Source: CAD feature listing. Evaluate the final solid. Frame: model axes, mm. Face numbers are marked on the shaded views. A direction names the side the tool comes from. Coordinates: 2 decimals unless noted, no trailing zeros. Write each loop counter-clockwise with the first axis right and the second up, starting at its lowest first coordinate (ties: lowest second). Pieces come first, ordered by that corner, then holes. Notation, with made-up numbers: (14.25, -21.5) -> (49.25, -21.5) arc R15 cw to (49.25, 7.5) -> close; hole circle Ø8 at (52.25, 83.5). An arc over 180 degrees is marked (long way). One line per item, written item: value. Start each with the question number.
1. Line query: line 1 (Z direction, x = 8, y = 120); line 2 (X direction, y = 14, z = -73); line 3 (Y direction, x = 83.5, z = -81). Output: solid intervals per line, ascending.
2. Section query B-B, the plane x = 58. Output: boundary loops of the cut face in (y, z).
3. Section query A-A, the plane y = 32.5. Output: boundary loops of the cut face in (x, z), and give its area (3 significant figures).
4. First-contact query: P1, Ø10, axis at x = 53.5, y = 24, coming from the -Z side (3 decimals); P2, Ø5, axis at x = 89.5, z = -89, coming from the +Y side; P3, Ø8, axis at y = 109.5, z = -16, coming from the -X side. Flat tips, straight axial feed; report the tip coordinate or a pass-through.
5. Section query C-C, the plane y = 80.5. Output: boundary loops of the cut face in (x, z).
6. Mould query, pull axis Y, two halves, no side actions, for the marked faces 4, 5 and 6. Classes: released by +Y, released by -Y, zero draft, split by the parting line, or undercut.
7. Access query for the marked faces 1, 2 and 3. Directions: +Z, -Z, +X, -X, +Y, -Y. A direction counts if a zero-diameter tool reaches every point of the face in a straight line with its end or side. Return the directions, or none.
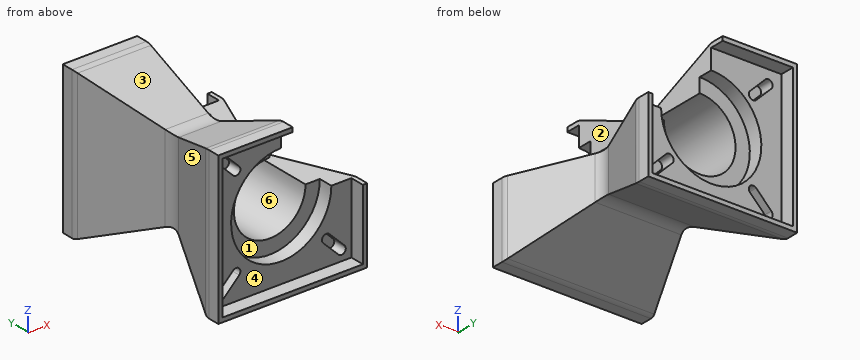
from build123d import *

# Parameters (mm, degrees)
SKETCH1_W           = 104
SKETCH1_H           = 104
BOSS_EXTRUDE1_DEPTH = 115
CUT_EXTRUDE1_DEPTH  = 187.70029459
SKETCH3_R           = 25
CUT_EXTRUDE2_DEPTH  = 187.70029459
CIRPATTERN1_COUNT   = 4
SKETCH4_R           = 35
CUT_EXTRUDE3_DEPTH  = 10
CUT_EXTRUDE4_START  = -10
SKETCH5_R           = 35
CUT_EXTRUDE4_DEPTH  = 10
FILLET2_R           = 15
SKETCH6_W           = 104
SKETCH6_H           = 104
SKETCH6_W_2         = 98
SKETCH6_H_2         = 98
BOSS_EXTRUDE2_DEPTH = 10
SKETCH7_W           = 104
SKETCH7_H           = 104
SKETCH7_W_2         = 98
SKETCH7_H_2         = 98
BOSS_EXTRUDE3_DEPTH = 10
CUT_EXTRUDE8_DEPTH  = 10
CUT_EXTRUDE9_DEPTH  = 10
FILLET3_R           = 10
SKETCH11_W          = 52
SKETCH11_H          = 52
CUT_EXTRUDE11_DEPTH = 200.642179912


with BuildPart() as part:
    # Sketch1 → Boss-Extrude1 (new body)
    with BuildSketch(Plane(origin=(0, 0, 0), x_dir=(1, 0, 0), z_dir=(0, 1, 0))):
        with Locations((52, 52)):
            Rectangle(SKETCH1_W, SKETCH1_H)
    extrude(amount=BOSS_EXTRUDE1_DEPTH)

    # Sketch2 → Cut-Extrude1 (cut, symmetric)
    with BuildSketch(Plane.XY):
        Polygon((229.074287939, 409.656557146), (104, 115), (79.592698068, 57.5), (104, 0), (229.074287939, -294.656557146), (869.280705191, -294.656557146), (869.280705191, 409.656557146), align=None)
    cut_extrude1 = extrude(amount=CUT_EXTRUDE1_DEPTH, both=True, mode=Mode.SUBTRACT)

    # Sketch3 → Cut-Extrude2 (cut, through all)
    with BuildSketch(Plane(origin=(0, 115, 0), x_dir=(1, 0, 0), z_dir=(0, 1, 0))):
        with Locations(Location((52, 52, 0), (0, 0, 270))):
            Circle(SKETCH3_R)
    cut_extrude2 = extrude(amount=-CUT_EXTRUDE2_DEPTH, mode=Mode.SUBTRACT)

    # CirPattern1: Cut-Extrude1, Cut-Extrude2 ×4 about axis
    cirpattern1_axis = Axis((52, 0, -52), (0, 1, 0))
    add([cut_extrude1.rotate(cirpattern1_axis, i * 360 / CIRPATTERN1_COUNT) for i in range(1, CIRPATTERN1_COUNT)], mode=Mode.SUBTRACT)
    add([cut_extrude2.rotate(cirpattern1_axis, i * 360 / CIRPATTERN1_COUNT) for i in range(1, CIRPATTERN1_COUNT)], mode=Mode.SUBTRACT)

    # Sketch4 → Cut-Extrude3 (cut)
    with BuildSketch(Plane(origin=(0, 115, 0), x_dir=(1, 0, 0), z_dir=(0, 1, 0))):
        with Locations(Location((52, 52, 0), (0, 0, 270))):
            Circle(SKETCH4_R)
    extrude(amount=-CUT_EXTRUDE3_DEPTH, mode=Mode.SUBTRACT)

    # Sketch5 → Cut-Extrude4 (cut)
    with BuildSketch(Plane.XZ.offset(CUT_EXTRUDE4_START)):
        with Locations(Location((52, -52, 0), (0, 0, 90))):
            Circle(SKETCH5_R)
    extrude(amount=CUT_EXTRUDE4_DEPTH, mode=Mode.SUBTRACT)

    # Fillet2
    fillet2_edges = [part.edges().sort_by_distance(p)[0] for p in [
        (79.592698068, 57.5, -52),
        (52, 57.5, -24.407301932),
        (24.407301932, 57.5, -52),
        (52, 57.5, -79.592698068),
    ]]
    fillet(fillet2_edges, radius=FILLET2_R)

    # Sketch6 → Boss-Extrude2 (add)
    with BuildSketch(Plane(origin=(0, 115, 0), x_dir=(1, 0, 0), z_dir=(0, 1, 0))):
        with Locations((52, 52)):
            Rectangle(SKETCH6_W, SKETCH6_H)
        with Locations((52, 52)):
            Rectangle(SKETCH6_W_2, SKETCH6_H_2, mode=Mode.SUBTRACT)
    extrude(amount=BOSS_EXTRUDE2_DEPTH)

    # Sketch7 → Boss-Extrude3 (add)
    with BuildSketch(Plane.XZ):
        with Locations((52, -52)):
            Rectangle(SKETCH7_W, SKETCH7_H)
        with Locations((52, -52)):
            Rectangle(SKETCH7_W_2, SKETCH7_H_2, mode=Mode.SUBTRACT)
    extrude(amount=BOSS_EXTRUDE3_DEPTH)

    # Sketch8 → Cut-Extrude8 (cut)
    with BuildSketch(Plane.XZ):
        with BuildLine():
            Line((85.587572106, -22.655068581), (96.194173824, -12.048466863))
            ThreePointArc((96.194173824, -12.048466863), (96.194173824, -7.805826176), (91.951533137, -7.805826176))
            Line((91.951533137, -7.805826176), (81.344931419, -18.412427894))
            ThreePointArc((81.344931419, -18.412427894), (81.344931419, -22.655068581), (85.587572106, -22.655068581))
        make_face()
        with BuildLine():
            Line((18.412427894, -81.344931419), (7.805826176, -91.951533137))
            ThreePointArc((7.805826176, -91.951533137), (7.805826176, -96.194173824), (12.048466863, -96.194173824))
            Line((12.048466863, -96.194173824), (22.655068581, -85.587572106))
            ThreePointArc((22.655068581, -85.587572106), (22.655068581, -81.344931419), (18.412427894, -81.344931419))
        make_face()
        with BuildLine():
            Line((22.655068581, -18.412427894), (12.048466863, -7.805826176))
            ThreePointArc((12.048466863, -7.805826176), (7.805826176, -7.805826176), (7.805826176, -12.048466863))
            Line((7.805826176, -12.048466863), (18.412427894, -22.655068581))
            ThreePointArc((18.412427894, -22.655068581), (22.655068581, -22.655068581), (22.655068581, -18.412427894))
        make_face()
        with BuildLine():
            Line((81.344931419, -85.587572106), (91.951533137, -96.194173824))
            ThreePointArc((91.951533137, -96.194173824), (96.194173824, -96.194173824), (96.194173824, -91.951533137))
            Line((96.194173824, -91.951533137), (85.587572106, -81.344931419))
            ThreePointArc((85.587572106, -81.344931419), (81.344931419, -81.344931419), (81.344931419, -85.587572106))
        make_face()
    extrude(amount=-CUT_EXTRUDE8_DEPTH, mode=Mode.SUBTRACT)

    # Sketch9 → Cut-Extrude9 (cut)
    with BuildSketch(Plane(origin=(0, 115, 0), x_dir=(1, 0, 0), z_dir=(0, 1, 0))):
        with BuildLine():
            Line((79.141990106, 83.384630793), (89.748591824, 93.991232511))
            ThreePointArc((89.748591824, 93.991232511), (93.991232511, 93.991232511), (93.991232511, 89.748591824))
            Line((93.991232511, 89.748591824), (83.384630793, 79.141990106))
            ThreePointArc((83.384630793, 79.141990106), (79.141990106, 79.141990106), (79.141990106, 83.384630793))
        make_face()
        with BuildLine():
            Line((83.384630793, 24.858009894), (93.991232511, 14.251408176))
            ThreePointArc((93.991232511, 14.251408176), (93.991232511, 10.008767489), (89.748591824, 10.008767489))
            Line((89.748591824, 10.008767489), (79.141990106, 20.615369207))
            ThreePointArc((79.141990106, 20.615369207), (79.141990106, 24.858009894), (83.384630793, 24.858009894))
        make_face()
        with BuildLine():
            Line((24.858009894, 20.615369207), (14.251408176, 10.008767489))
            ThreePointArc((14.251408176, 10.008767489), (10.008767489, 10.008767489), (10.008767489, 14.251408176))
            Line((10.008767489, 14.251408176), (20.615369207, 24.858009894))
            ThreePointArc((20.615369207, 24.858009894), (24.858009894, 24.858009894), (24.858009894, 20.615369207))
        make_face()
        with BuildLine():
            Line((20.615369207, 79.141990106), (10.008767489, 89.748591824))
            ThreePointArc((10.008767489, 89.748591824), (10.008767489, 93.991232511), (14.251408176, 93.991232511))
            Line((14.251408176, 93.991232511), (24.858009894, 83.384630793))
            ThreePointArc((24.858009894, 83.384630793), (24.858009894, 79.141990106), (20.615369207, 79.141990106))
        make_face()
    extrude(amount=-CUT_EXTRUDE9_DEPTH, mode=Mode.SUBTRACT)

    # Fillet3
    fillet3_edges = [part.edges().sort_by_distance(p)[0] for p in [
        (104, 115, -52),
        (52, 115, -104),
        (0, 115, -52),
        (52, 0, -104),
        (104, 0, -52),
        (52, 0, 0),
        (0, 0, -52),
        (52, 115, 0),
    ]]
    fillet(fillet3_edges, radius=FILLET3_R)

    # Sketch11 → Cut-Extrude11 (cut, through all)
    with BuildSketch(Plane(origin=(0, 125, 0), x_dir=(1, 0, 0), z_dir=(0, 1, 0))):
        with Locations((78, 26)):
            Rectangle(SKETCH11_W, SKETCH11_H)
    extrude(amount=-CUT_EXTRUDE11_DEPTH, mode=Mode.SUBTRACT)


solid = part.part
Computed values:
1. line 1: z = -104 to -101, -3 to 0
1. line 2: x = 5.94 to 38.44, 65.56 to 98.06
1. line 3: y = 10 to 48.29, 66.71 to 105
2. outline: (-10, -104) -> (-2.03, -104) arc R10 ccw to (1.87, -103.21) -> (51.64, -82.08) arc R15 cw to (63.36, -82.08) -> (113.13, -103.21) arc R10 ccw to (117.03, -104) -> (125, -104) -> (125, -101) -> (115, -101) -> (115, -86.48) -> (105, -86.48) -> (105, -76.27) -> (10, -76.27) -> (10, -86.48) -> (0, -86.48) -> (0, -101) -> (-10, -101) -> close
3. outline: (13.8, -90.2) -> (90.2, -90.2) -> (90.2, -52) -> (77, -52) arc R25 cw (long way) to (52, -27) -> (52, -13.8) -> (13.8, -13.8) -> close
3. area: 2,910 mm²
4. P1: stops at z = -95.935
4. P2: stops at y = 105
4. P3: stops at x = 0.65
5. outline: (14.64, -89.36) -> (89.36, -89.36) -> (89.36, -52) -> (77, -52) arc R25 cw (long way) to (52, -27) -> (52, -14.64) -> (14.64, -14.64) -> close
6. face 4: released by -Y
6. face 5: undercut
6. face 6: zero draft
7. face 1: -Y
7. face 2: +Z, +X, +Y, -Y
7. face 3: +Z, +X, -X
